Geometry: final body of the model. Coordinates: model frame, mm. Face numbers are marked on the shaded views. A direction names the side the tool comes from. Round coordinates to 2 decimals unless told otherwise and drop trailing zeros. Order: outer loops, then holes, each group sorted by start corner. A loop starts at its lowest first (then second) coordinate and runs counter-clockwise, first axis right, second up. Notation, with made-up numbers: M 38.5,-3.5 L 84.5,-3.5 A14 cw 84.5,13.5 Z; hole C 32,-18.5 d3. An arc over 180 degrees is marked long. Return JSON: item names as keys, results as strings. Group by question number.
Q1. Cut plane B-B on y = 16.5. Output: boundary loops of the cut face in (x, z).
Q2. Cut plane A-A on x = -2. Count the separate pieces of the cut face and the enclosed holes in it, and give its area (3 significant figures).
Q3. Cut plane D-D on y = 3. Output: boundary loops of the cut face in (x, z).
Q4. Access query for the marked faces 1, 2, 3, 4 and 5. Directions: +Z, -Z, +X, -X, +Y, -Y. A direction counts if a zero-diameter tool reaches every point of the face in a straight line with its end or side. Return the directions, or none.
Q5. Contact query for flat-ended pins moving along their axis: pin 1 (6 mm diameter, centred on x = 0, z = -10.5, fed in from -Y); pin 2 (5 mm diameter, centred on x = 10, y = 5, fed in from -Z); pin 3 (2 mm diameter, centred on x = -5.5, y = 32, fed in from +Z); pin 4 (1.5 mm diameter, centred on x = -15, y = 6.5, fed in from +Z). Output: stop coordinate, or through.
Q6. Mould query, pull axis X, two halves, no side actions, for the marked faces 6, 7, 8 and 9. Classes: released by +X, released by -X, zero draft, split by the parting line, or undercut.
Q7. Ray query, probe 1 along Z at (x, y) = (-5.5, 28); probe 2 along X at (y, z) = (30.5, -10.25); probe 3 along Z at (x, y) = (-4.5, 26). Return the intervals inside material, ascending.
```python
from build123d import *

# Parameters (mm, degrees)
PAD_DEPTH            = 20
SKETCH001_W          = 37
SKETCH001_H          = 5
PAD001_DEPTH         = 6.5
SKETCH003_W          = 27
SKETCH003_H          = 28.5
POCKET001_DEPTH      = 3.5
SKETCH004_R          = 1.65
POCKET002_DEPTH      = 20.001
SKETCH005_R          = 3.5
POCKET003_DEPTH      = 14.5
POCKET004_DEPTH      = 18.501
POCKET004_DEPTH_BACK = -18.501
PAD002_DEPTH         = 18.5
POCKET_DEPTH         = 13.5
SKETCH008_W          = 2
SKETCH008_H          = 5
POCKET005_DEPTH      = 18.501
POCKET005_DEPTH_BACK = -18.501
FILLET_R             = 3
FILLET001_R          = 9.99
FILLET002_R          = 19.99
FILLET003_R          = 2


with BuildPart() as part:
    # Sketch → Pad (new body)
    with BuildSketch(Plane.XY):
        Polygon((-18.5, 0), (-18.5, 38.5), (18.5, 38.5), (18.5, 0), (13.5, 0), (13.5, 23.5), (-13.5, 23.5), (-13.5, 0), align=None)
    extrude(amount=-PAD_DEPTH)

    # Sketch001 → Pad001 (join)
    with BuildSketch(Plane.XY):
        with Locations((0, 26)):
            Rectangle(SKETCH001_W, SKETCH001_H)
    extrude(amount=PAD001_DEPTH)

    # Sketch003 → Pocket001 (cut)
    with BuildSketch(Plane.XY):
        with Locations((0, 14.25)):
            Rectangle(SKETCH003_W, SKETCH003_H)
    extrude(amount=POCKET001_DEPTH, mode=Mode.SUBTRACT)

    # Sketch004 → Pocket002 (cut, through all)
    with BuildSketch(Plane.XY):
        with Locations((-6.5, 30.5)):
            Circle(SKETCH004_R)
        with Locations((6.5, 30.5)):
            Circle(SKETCH004_R)
    extrude(amount=-POCKET002_DEPTH, mode=Mode.SUBTRACT)

    # Sketch005 → Pocket003 (cut)
    with BuildSketch(Plane.XY):
        with Locations((-6.5, 30.5)):
            Circle(SKETCH005_R)
        with Locations((6.5, 30.5)):
            Circle(SKETCH005_R)
    extrude(amount=-POCKET003_DEPTH, mode=Mode.SUBTRACT)

    # Sketch006 → Pocket004 (cut, two sides)
    with BuildSketch(Plane.YZ) as pocket004_sk:
        Polygon((28.5, 0), (43.5, 0), (43.5, -20), align=None)
    extrude(amount=-POCKET004_DEPTH, mode=Mode.SUBTRACT)
    extrude(pocket004_sk.sketch, amount=-POCKET004_DEPTH_BACK, mode=Mode.SUBTRACT)

    # Sketch007 → Pad002 (join, symmetric)
    with BuildSketch(Plane.YZ):
        Polygon((13.5, 0), (23.5, 0), (23.5, 6.5), align=None)
    extrude(amount=PAD002_DEPTH, both=True)

    # Sketch007 → Pocket (cut, symmetric)
    with BuildSketch(Plane.YZ):
        Polygon((13.5, 0), (23.5, 0), (23.5, 6.5), align=None)
    extrude(amount=POCKET_DEPTH, both=True, mode=Mode.SUBTRACT)

    # Sketch008 → Pocket005 (cut, two sides)
    with BuildSketch(Plane.YZ) as pocket005_sk:
        with Locations((25.5, -10)):
            Rectangle(SKETCH008_W, SKETCH008_H)
    extrude(amount=-POCKET005_DEPTH, mode=Mode.SUBTRACT)
    extrude(pocket005_sk.sketch, amount=-POCKET005_DEPTH_BACK, mode=Mode.SUBTRACT)

    # Fillet
    fillet_edges = [part.edges().sort_by_distance(p)[0] for p in [
        (18.5, 24.5, -10),
        (-18.5, 24.5, -10),
        (18.5, 26.5, -10),
        (-18.5, 26.5, -10),
    ]]
    fillet(fillet_edges, radius=FILLET_R)

    # Fillet001
    fillet001_edges = [part.edges().sort_by_distance(p)[0] for p in [
        (16, 28.5, 0),
        (-16, 28.5, 0),
    ]]
    fillet(fillet001_edges, radius=FILLET001_R)

    # Fillet002
    fillet002_edges = [part.edges().sort_by_distance(p)[0] for p in [
        (0, 38.5, -13.333333),
    ]]
    fillet(fillet002_edges, radius=FILLET002_R)

    # Fillet003
    fillet003_edges = [part.edges().sort_by_distance(p)[0] for p in [
        (18.5, 37.474179, -13.675274),
        (-18.5, 37.474179, -13.675274),
        (18.5, 0, -10),
        (13.5, 0, -10),
        (-13.5, 0, -10),
        (-18.5, 0, -10),
    ]]
    fillet(fillet003_edges, radius=FILLET003_R)


solid = part.part
```
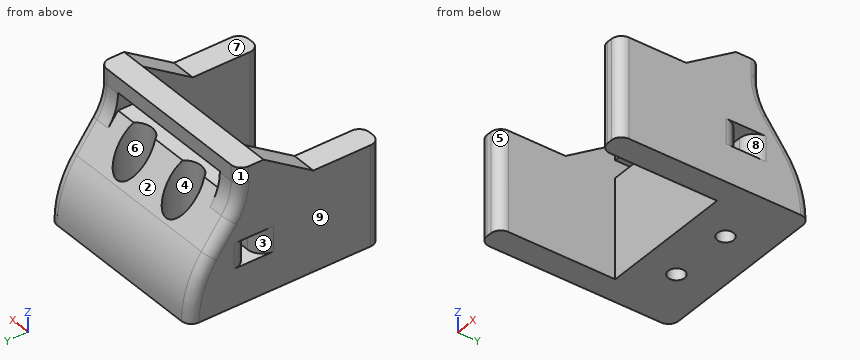
Result sheet:
{
 "1": {"outline": "M -18.5,-20 L -13.5,-20 L -13.5,1.95 L -18.5,1.95 Z; M 13.5,-20 L 18.5,-20 L 18.5,1.95 L 13.5,1.95 Z"},
 "2": {"separate pieces": "2", "enclosed holes": "1", "area": "234 mm²"},
 "3": {"outline": "M -18.5,-20 L -13.5,-20 L -13.5,0 L -18.5,0 Z; M 13.5,-20 L 18.5,-20 L 18.5,0 L 13.5,0 Z"},
 "4": {"face 1": "+Z, -X, +Y", "face 2": "+Z, +Y", "face 3": "-X", "face 4": "none", "face 5": "+Z, -Z, -Y"},
 "5": {"pin 1": "stops at y = 23.5", "pin 2": "passes through", "pin 3": "stops at z = -14.5", "pin 4": "stops at z = 0"},
 "6": {"face 6": "undercut", "face 7": "zero draft", "face 8": "released by +X", "face 9": "released by -X"},
 "7": {"probe 1": "z = -20 to -14.5, 3.5 to 6.5", "probe 2": "x = -18.5 to -10, -3 to 3, 10 to 18.5", "probe 3": "z = -20 to -12.5, -7.5 to 0, 3.5 to 6.5"}
}
